Part model, mm, in its own coordinate system. Face numbers are marked on the shaded views. A direction names the side the tool comes from. Coordinates: 2 decimals unless noted, no trailing zeros. Loops run counter-clockwise (first coordinate to the right, second up) from the corner with the lowest first, then second, coordinate; pieces in that order, holes last. Notation, with made-up numbers: (42.25, -24.5) -> (89.25, -24.5) arc R32 ccw to (89.25, 13.5) -> close; hole circle Ø6 at (-39, 23.5). An arc over 180 degrees is marked (long way). One line per item, written item: value. Start each with the question number.
from build123d import *

# Parameters (mm, degrees)
BOSS_EXTRUDE1_DEPTH = 3
BOSS_EXTRUDE2_DEPTH = 64
SKETCH3_R           = 90
BOSS_EXTRUDE4_DEPTH = 19


with BuildPart() as part:
    # Sketch1 → Boss-Extrude1 (new body)
    with BuildSketch(Plane.XY):
        with BuildLine():
            Line((-131.94247797, 0), (238.05752203, 0))
            ThreePointArc((238.05752203, 0), (328.05752203, 90), (238.05752203, 180))
            Line((238.05752203, 180), (-131.94247797, 180))
            Line((-131.94247797, 180), (-131.94247797, 0))
        make_face()
    extrude(amount=BOSS_EXTRUDE1_DEPTH)

    # Sketch2 → Boss-Extrude2 (add)
    # profile 1 of 4: a face of its own
    with BuildSketch(Plane.XY.offset(3)):
        Polygon((203.021580666, 54.507604342), (176.500529327, 40.484985617), (162.477910603, 67.006036956), (188.998961942, 81.02865568), align=None)
        Polygon((177.750372588, 44.539352624), (166.532277609, 65.756193695), (187.74911868, 76.974288674), (198.967213659, 55.757447603), align=None, mode=Mode.SUBTRACT)
    # profile 2 of 4: a face of its own
    with BuildSketch(Plane.XY.offset(3)):
        Polygon((287.572536413, 28.443007297), (261.051485074, 14.420388572), (247.02886635, 40.941439911), (273.549917689, 54.964058635), align=None)
        Polygon((262.301328336, 18.474755579), (251.083233356, 39.69159665), (272.300074427, 50.909691629), (283.518169407, 29.692850558), align=None, mode=Mode.SUBTRACT)
    # profile 3 of 4: a face of its own
    with BuildSketch(Plane.XY.offset(3)):
        Polygon((299.614514734, 139.515014383), (313.637133458, 112.993963044), (287.116082119, 98.97134432), (273.093463395, 125.492395658), align=None)
        Polygon((309.582766452, 114.243806305), (288.365925381, 103.025711326), (277.147830401, 124.242552397), (298.364671472, 135.460647376), align=None, mode=Mode.SUBTRACT)
    # profile 4 of 4: a face of its own
    with BuildSketch(Plane.XY.offset(3)):
        Polygon((188.542507648, 151.556992703), (215.063558987, 165.579611428), (229.086177711, 139.058560089), (202.565126372, 125.035941365), align=None)
        Polygon((203.814969633, 129.090308371), (192.596874654, 150.307149442), (213.813715725, 161.525244421), (225.031810705, 140.30840335), align=None, mode=Mode.SUBTRACT)
    extrude(amount=BOSS_EXTRUDE2_DEPTH)

    # Sketch3 → Boss-Extrude4 (add)
    with BuildSketch(Plane.XY.offset(67)):
        with Locations((238.05752203, 90)):
            Circle(SKETCH3_R)
    extrude(amount=BOSS_EXTRUDE4_DEPTH)


solid = part.part
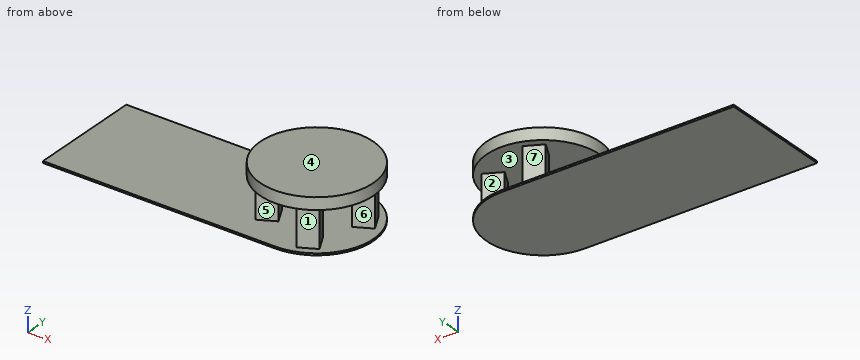
1) Pin check, flat tips, straight feed: pin 1 Ø8 at (y, z) = (131, 65.5) entering from -X; pin 2 Ø6 at (x, y) = (-84.5, 76) entering from +Z; pin 3 Ø5 at (y, z) = (139.5, 28) entering from -X. Stop position of each tip, or through.
2) Slice it at C-C (x = 128.5). Give the cut face in (y, z), then the cut area to 3 significant figures.
3) Slice it at A-A (y = 90). Give the cut face in (x, z).
4) Probe line 1 (Z direction, x = 191.5, y = 124); line 2 (Y direction, x = 198, z = 44); line 3 (X direction, y = 136, z = 25). List the from-to ranges inside material, lowest first. Write a range as from..to.
5) Slice it at B-B (z = 78.5). Give the cut face in (x, y).
6) Tool access for the marked faces 1, 2, 3 and 4: list every direction of +Z, -Z, +X, -X, +Y, -Y with a clear straight run to the whole face (end or side of a thin tool).
7) Pull direction X, two halves, no side cores. Call the marked faces 5, 6 and 7: +X half, -X half, draft (parallel to the pull), parting line (faces both ways), or undercut.
Check sheet entries:
1. pin 1: stops at x = 156.15
1. pin 2: stops at z = 3
1. pin 3: stops at x = 193.6
2. outline: (0, 0) -> (180, 0) -> (180, 3) -> (0, 3) -> close
2. area: 540 mm^2
3. outline: (-131.94, 0) -> (328.06, 0) -> (328.06, 3) -> (-131.94, 3) -> close; (148.06, 67) -> (328.06, 67) -> (328.06, 86) -> (148.06, 86) -> close
4. line 1: z = 0..3, 67..86
4. line 2: y = 51.85..55.25, 57.59..64, 133.67..140.09, 153.16..156.56
4. line 3: x = 196.77..200.16, 216.88..223.3, 292.97..301.47
5. outline: circle Ø180 at (238.06, 90)
6. face 1: +X, -Y
6. face 2: +Y
6. face 3: none
6. face 4: +Z, +X, -X, +Y, -Y
7. face 5: undercut
7. face 6: +X half
7. face 7: -X half
